Verification items for this drawing (mm, ordinates from the low corner). A direction names the side the tool comes from. Coordinates: 2 decimals unless noted, no trailing zeros. Write each loop counter-clockwise with the first axis right and the second up, starting at its lowest first coordinate (ties: lowest second). Pieces come first, ordered by that corner, then holes. Notation, with made-up numbers: M 18,2.25 L 55,2.25 A23 ccw 55,19.25 Z; hole C 34,8 d9. An arc over 180 degrees is marked long. Put each result on its own line as item: value. Start each with the question number.
1) Scan lines: line 1 along X through (y, z) = (7.5, 0.7) (1 decimal); line 2 along Y through (x, z) = (5.75, 0.45) (1 decimal); line 3 along Z through (x, y) = (8.25, 15.25). Record each from-to range of solid material in increasing order.
2) Set-up check for the marked faces 1, 2 and 3: record each of +Z, -Z, +X, -X, +Y, -Y from which the full face is reachable in a straight line by a thin tool's end or side.
3) Cross-section at C-C on y = 7.5. Count the separate pieces of the cut face and the enclosed holes in it.
4) Gauge pin test, flat end, axial feed: pin 1 (2 mm diameter, centred on x = 5.26, y = 8.09, fed in from +Z). Record the tip position at first contact, or that the pin passes through.
5) Mould release check, pull along X, two halves, no side actions. Record for the marked faces 4, 5, 6 and 7: released by +X, released by -X, zero draft, split by the parting line, or undercut.
6) Cross-section at D-D on z = 0.95. Record the cut outline in (x, y), plus the area to 3 significant figures.
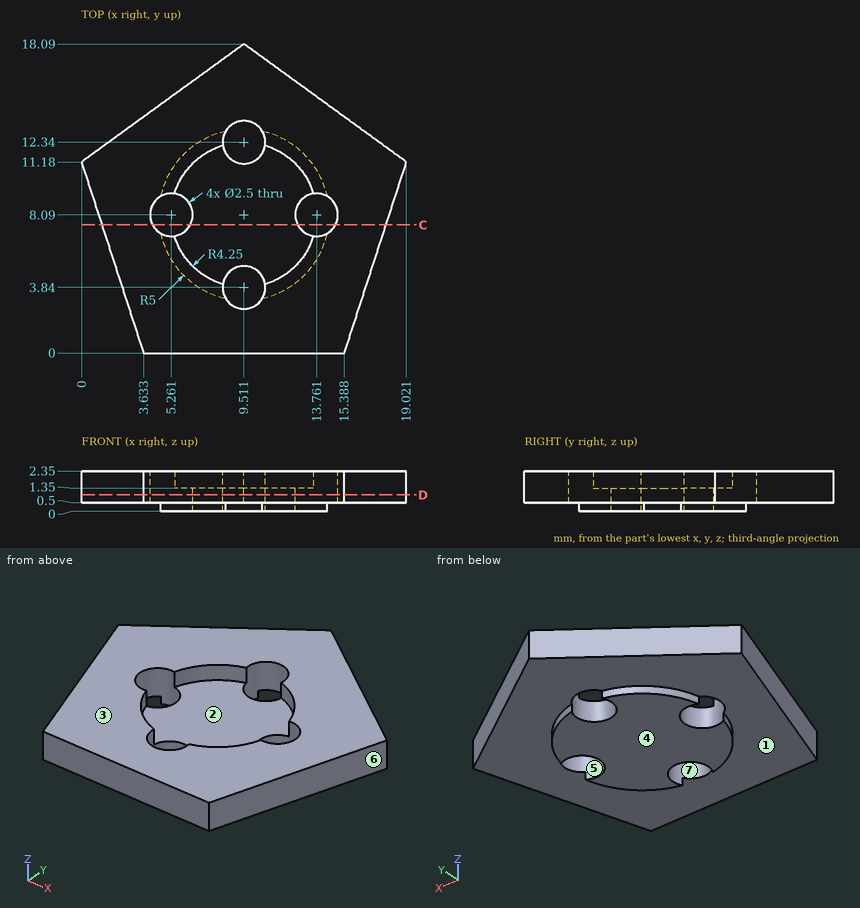
Answer key:
1. line 1: x = 1.2 to 4.2, 6.4 to 12.7, 14.9 to 17.8
1. line 2: y = 4.8 to 6.9, 9.2 to 11.4
1. line 3: z = 0.5 to 2.35
2. face 1: -Z
2. face 2: +Z
2. face 3: +Z, +X, -X, +Y, -Y
3. separate pieces: 3
3. enclosed holes: 0
4. pin 1: passes through
5. face 4: zero draft
5. face 5: undercut
5. face 6: released by +X
5. face 7: undercut
6. outline: M 0,11.18 L 3.63,0 L 15.39,0 L 19.02,11.18 L 9.51,18.09 Z; hole C 5.26,8.09 d2.5; hole C 9.51,3.84 d2.5; hole C 9.51,12.34 d2.5; hole C 13.76,8.09 d2.5
6. area: 218 mm²
